Can you work these out from the model? Positions are in its coordinate system, mm. Face numbers are marked on the shaded views. A direction names the side the tool comes from. Round coordinates to 2 decimals unless told otherwise and drop trailing zeros. Loops run counter-clockwise (first coordinate to the right, second up) from the corner with the lowest first, then second, coordinate; pieces in that order, holes last. Notation, with made-up numbers: (14, 53) -> (47, 53) arc R14 ccw to (47, 79) -> close; hole circle Ø10 at (-31.5, -14.5). An arc over 180 degrees is marked (long way). Answer as a JSON object with one key per item and string values.
```python
from build123d import *

# Parameters (mm, degrees)
F0_R     = 3.175
F1_DEPTH = 25.4
F2_W     = 25.4
F2_H     = 10.16
F3_DEPTH = 25.4
F5_DEPTH = 25.4
F4_R     = 3.175
F6_DEPTH = 7.62
F7_DEPTH = 25.4


with BuildPart() as f1:
    # F0 (on Front) → F1 (new body)
    with BuildSketch(Plane.XZ):
        with BuildLine():
            Line((38.1, 12.7), (-38.1, 12.7))
            ThreePointArc((-38.1, 12.7), (-50.8, 0), (-38.1, -12.7))
            Line((-38.1, -12.7), (38.1, -12.7))
            Line((38.1, -12.7), (38.1, 12.7))
        make_face()
        with Locations((-38.1, 0)):
            Circle(F0_R, mode=Mode.SUBTRACT)
    extrude(amount=F1_DEPTH)

    # F2 (on face) → F3 (join)
    with BuildSketch(Plane.YZ.offset(38.1)):
        with Locations((-12.7, 0)):
            Rectangle(F2_W, F2_H)
    extrude(amount=F3_DEPTH)

    # F4 (on face) → F5 (cut)
    with BuildSketch(Plane.XY.offset(5.08)):
        with BuildLine():
            ThreePointArc((50.8, 0), (59.7802561211, -3.7197438789), (63.5, -12.7))
            Line((63.5, -12.7), (63.5, 0))
            Line((63.5, 0), (50.8, 0))
        make_face()
        with BuildLine():
            Line((63.5, -25.4), (63.5, -12.7))
            ThreePointArc((63.5, -12.7), (59.7802561211, -21.6802561211), (50.8, -25.4))
            Line((50.8, -25.4), (63.5, -25.4))
        make_face()
    extrude(amount=-F5_DEPTH, mode=Mode.SUBTRACT)

    # F4 (on face) → F6 (join)
    with BuildSketch(Plane.XY.offset(5.08)):
        with Locations((50.8, -12.7)):
            Circle(F4_R)
    extrude(amount=F6_DEPTH)

    # F7 (add): a face of the model
    f7_faces = [f1.faces().sort_by_distance(p)[0] for p in [
        (50.8, -12.7, 12.7),
    ]]
    extrude(f7_faces, amount=-F7_DEPTH)


solid = f1.part
```
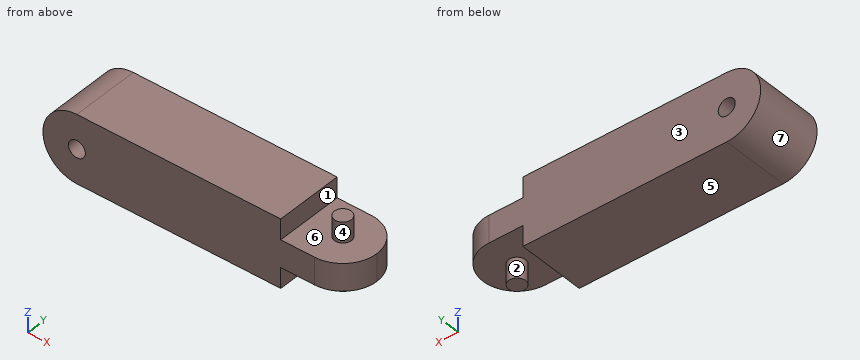
Q1. I want a section at A-A, the plane y = -20.25. Write out the boundary of the cut face in (x, z) (3 decimals), then the cut area to 3 significant figures.
Determined:
{"outline": "(-38.1, -12.7) -> (38.1, -12.7) -> (38.1, -5.08) -> (61.012, -5.08) -> (61.012, 5.08) -> (38.1, 5.08) -> (38.1, 12.7) -> (-38.1, 12.7) arc R12.7 ccw to start; hole circle Ø6.35 at (-38.1, 0)", "area": "2,390 mm²"}
Q2. I want a section at C-C, the plane y = -8.25. Write out the boundary of the cut face in (x, z) (3 decimals).
Determined:
{"outline": "(-38.1, -12.7) -> (38.1, -12.7) -> (38.1, -5.08) -> (62.695, -5.08) -> (62.695, 5.08) -> (38.1, 5.08) -> (38.1, 12.7) -> (-38.1, 12.7) arc R12.7 ccw to start; hole circle Ø6.35 at (-38.1, 0)"}
Q3. I want a section at B-B, the plane z = 7.5. Write out the boundary of the cut face in (x, y) (3 decimals).
Determined:
{"outline": "(-48.349, -25.4) -> (38.1, -25.4) -> (38.1, 0) -> (-48.349, 0) -> close; circle Ø6.35 at (50.8, -12.7)"}
Q4. On a 3-axis mill with a long thin cutter (end or side, diameter ignored), from which of +Z, -Z, +X, -X, +Y, -Y can I reach the whole of each face in a straight line? I mean the marked faces 1, 2 and 3. Say none if no direction works.
Determined:
{"face 1": "+Z, +Y, -Y", "face 2": "-Z", "face 3": "+Z, -Z, +X, -X, +Y"}
Q5. I'm going to push flat-ended pins straight in: pin 1 (4 mm diameter, centred on y = -11.5, z = -6, fed in from -X); pin 2 (12 mm diameter, centred on x = 29, z = -5, fed in from +Y); pin 3 (4 mm diameter, centred on y = -7, z = 3.5, fed in from -X); pin 4 (2 mm diameter, centred on y = -20, z = 4.5, fed in from +X). Where does each tip first touch, or does it pass through?
Determined:
{"pin 1": "x = -50.15", "pin 2": "y = 0", "pin 3": "x = -50.71", "pin 4": "x = 61.83"}
Q6. We'd pull the mould along X, two halves only. Please class the marked faces 4, 5, 6 and 7: pulls with the +X half, pulls with the -X half, needs draft (parallel to the pull), parting line crosses it, or undercut.
Determined:
{"face 4": "undercut", "face 5": "needs draft", "face 6": "undercut", "face 7": "pulls with the -X half"}
Q7. If I drill on L1, parallel to Z at x = -38.1, y = -16.25 (3 decimals); L2, parallel to X at y = -19, z = -1.25; L3, parallel to X at y = -14.5, z = 9.75, over which ranges is the centre line in solid material (lowest first)? Write a range as [from, to].
Determined:
{"L1": "[-12.7, -3.175], [3.175, 12.7]", "L2": "[-50.74, -41.02], [-35.18, 61.83]", "L3": "[-46.24, 38.1], [48.18, 53.42]"}
